Check sheet for the modelled part. Datum: model origin and axes. Units: mm. A direction names the side the tool comes from. Coordinates: 2 decimals unless noted, no trailing zeros. Write each loop counter-clockwise with the first axis right and the second up, starting at its lowest first coordinate (ties: lowest second). Pieces come first, ordered by that corner, then holes. Notation, with made-up numbers: (35.5, -16.75) -> (87.5, -16.75) arc R8 ccw to (87.5, -10.75) -> close; hole circle Ø8 at (31, 26). An arc over 180 degrees is marked (long way). Put each result on its own line as item: value.
```python
from build123d import *

# Parameters (mm, degrees)
F0_W     = 1104.9
F0_H     = 76.2
F1_DEPTH = 10.31875
F2_W     = 9.525
F2_H     = 20.6375
F3_DEPTH = 47.625
F4_W     = 9.525
F4_H     = 20.6375
F5_DEPTH = 47.625
F6_W     = 1104.9
F6_H     = 7.9375
F7_DEPTH = 9.525


with BuildPart() as f1:
    # F0 (on Front) → F1 (new body, symmetric)
    with BuildSketch(Plane.XZ):
        Rectangle(F0_W, F0_H)
    extrude(amount=F1_DEPTH, both=True)

    # F2 (on face) → F3 (join)
    with BuildSketch(Plane.YZ.offset(552.45)):
        with Locations((0, 18.25625)):
            Rectangle(F2_W, F2_H)
        with Locations((0, -18.25625)):
            Rectangle(F2_W, F2_H)
    extrude(amount=F3_DEPTH)

    # F4 (on face) → F5 (join)
    with BuildSketch(Plane(origin=(-552.45, 0, 0), x_dir=(0, -1, 0), z_dir=(-1, 0, 0))):
        with Locations((0, -18.25625)):
            Rectangle(F4_W, F4_H)
        with Locations((0, 18.25625)):
            Rectangle(F4_W, F4_H)
    extrude(amount=F5_DEPTH)

    # F6 (on face) → F7 (cut)
    with BuildSketch(Plane(origin=(0, 0, -38.1), x_dir=(1, 0, 0), z_dir=(0, 0, -1))):
        Rectangle(F6_W, F6_H)
    extrude(amount=-F7_DEPTH, mode=Mode.SUBTRACT)


solid = f1.part
```
Q1. Depth check by flat-ended pin: P1, Ø22.5, axis at x = 575, z = -13.5, coming from the -Y side; P2, Ø22.5, axis at x = 583, z = 22, coming from the +Y side; P3, Ø3, axis at x = -577.5, y = -1, coming from the +Z side (3 decimals). Enter the tip coordinate at first touch or a pass-through.
Recorded:
P1: stops at y = -4.76
P2: stops at y = 4.76
P3: stops at z = 28.575
Q2. Tool access check on faces 5 (the flat face through (-576, -4.762, -18)), 6 (the flat face through (576, 4.762, -18)), 7 (the flat face through (576, -4.762, 18)). Record the directions out of +Z, -Z, +X, -X, +Y, -Y that give a thin tool (end or side, any length) a straight path to the whole face; none if there is none.
Recorded:
face 5: +Z, -Z, -X, -Y
face 6: +Z, -Z, +X, +Y
face 7: +Z, -Z, +X, -Y
Q3. Mould release check, pull along Z, two halves, no side actions. Record for faces 1 (the flat face through (-8, 0, 38.1)), 2 (the flat face through (-552.45, 0, -1)), 3 (the flat face through (-576, 4.762, -18)), 4 (the flat face through (552.45, 0, -1)): released by +Z, released by -Z, zero draft, split by the parting line, or undercut.
Recorded:
face 1: released by +Z
face 2: undercut
face 3: zero draft
face 4: undercut
Q4. Cross-section at A-A (x = 155.5). Record the cut outline in (y, z) (3 decimals).
Recorded:
outline: (-10.319, -38.1) -> (-3.969, -38.1) -> (-3.969, -28.575) -> (3.969, -28.575) -> (3.969, -38.1) -> (10.319, -38.1) -> (10.319, 38.1) -> (-10.319, 38.1) -> close
Q5. Material ranges on line 1 along Y through (x, z) = (-502, -34.5); line 2 along X through (y, z) = (-9.5, -19.5); line 3 along Z through (x, y) = (349.5, 2.25) (3 decimals), recorded low to high.
Recorded:
line 1: y = -10.32 to -3.97, 3.97 to 10.32
line 2: x = -552.45 to 552.45
line 3: z = -28.575 to 38.1
